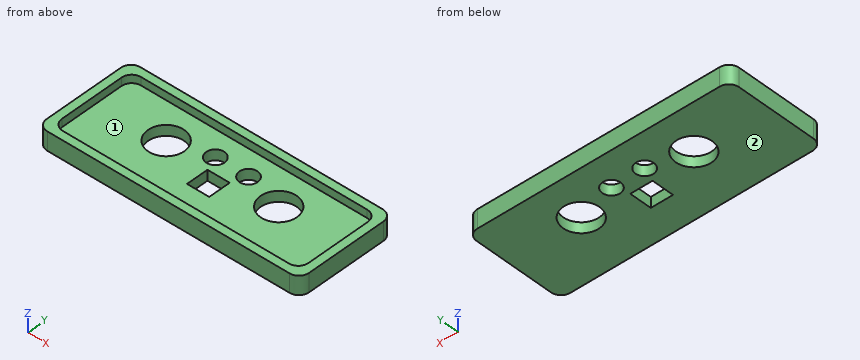
```python
from build123d import *

# Parameters (mm, degrees)
F1_DEPTH = 3.302
F2_DEPTH = 2.54
F3_R     = 5.715
F3_W     = 6.985
F3_H     = 6.985
F3_R_2   = 2.8702
F4_DEPTH = 3.303


with BuildPart() as f1:
    # F0 (on Top) → F1 (new body)
    with BuildSketch(Plane.XY):
        with BuildLine():
            Line((86.51892, -3.862933), (10.31892, -3.862933))
            ThreePointArc((10.31892, -3.862933), (8.073856, -4.792869), (7.14392, -7.037933))
            Line((7.14392, -7.037933), (7.14392, -32.437933))
            ThreePointArc((7.14392, -32.437933), (8.073856, -34.682997), (10.31892, -35.612933))
            Line((10.31892, -35.612933), (86.51892, -35.612933))
            ThreePointArc((86.51892, -35.612933), (88.763984, -34.682997), (89.69392, -32.437933))
            Line((89.69392, -32.437933), (89.69392, -7.037933))
            ThreePointArc((89.69392, -7.037933), (88.763984, -4.792869), (86.51892, -3.862933))
        make_face()
        with BuildLine():
            Line((83.97892, -33.072933), (12.85892, -33.072933))
            ThreePointArc((12.85892, -33.072933), (10.613856, -32.142997), (9.68392, -29.897933))
            Line((9.68392, -29.897933), (9.68392, -9.577933))
            ThreePointArc((9.68392, -9.577933), (10.613856, -7.332869), (12.85892, -6.402933))
            Line((12.85892, -6.402933), (83.97892, -6.402933))
            ThreePointArc((83.97892, -6.402933), (86.223984, -7.332869), (87.15392, -9.577933))
            Line((87.15392, -9.577933), (87.15392, -29.897933))
            ThreePointArc((87.15392, -29.897933), (86.223984, -32.142997), (83.97892, -33.072933))
        make_face(mode=Mode.SUBTRACT)
        with BuildLine():
            ThreePointArc((9.68392, -29.897933), (10.613856, -32.142997), (12.85892, -33.072933))
            Line((12.85892, -33.072933), (83.97892, -33.072933))
            ThreePointArc((83.97892, -33.072933), (86.223984, -32.142997), (87.15392, -29.897933))
            Line((87.15392, -29.897933), (87.15392, -9.577933))
            ThreePointArc((87.15392, -9.577933), (86.223984, -7.332869), (83.97892, -6.402933))
            Line((83.97892, -6.402933), (12.85892, -6.402933))
            ThreePointArc((12.85892, -6.402933), (10.613856, -7.332869), (9.68392, -9.577933))
            Line((9.68392, -9.577933), (9.68392, -29.897933))
        make_face()
    extrude(amount=-F1_DEPTH)

    # F0 (on Top) → F2 (join)
    with BuildSketch(Plane.XY):
        with BuildLine():
            Line((86.51892, -3.862933), (10.31892, -3.862933))
            ThreePointArc((10.31892, -3.862933), (8.073856, -4.792869), (7.14392, -7.037933))
            Line((7.14392, -7.037933), (7.14392, -32.437933))
            ThreePointArc((7.14392, -32.437933), (8.073856, -34.682997), (10.31892, -35.612933))
            Line((10.31892, -35.612933), (86.51892, -35.612933))
            ThreePointArc((86.51892, -35.612933), (88.763984, -34.682997), (89.69392, -32.437933))
            Line((89.69392, -32.437933), (89.69392, -7.037933))
            ThreePointArc((89.69392, -7.037933), (88.763984, -4.792869), (86.51892, -3.862933))
        make_face()
        with BuildLine():
            Line((83.97892, -33.072933), (12.85892, -33.072933))
            ThreePointArc((12.85892, -33.072933), (10.613856, -32.142997), (9.68392, -29.897933))
            Line((9.68392, -29.897933), (9.68392, -9.577933))
            ThreePointArc((9.68392, -9.577933), (10.613856, -7.332869), (12.85892, -6.402933))
            Line((12.85892, -6.402933), (83.97892, -6.402933))
            ThreePointArc((83.97892, -6.402933), (86.223984, -7.332869), (87.15392, -9.577933))
            Line((87.15392, -9.577933), (87.15392, -29.897933))
            ThreePointArc((87.15392, -29.897933), (86.223984, -32.142997), (83.97892, -33.072933))
        make_face(mode=Mode.SUBTRACT)
    extrude(amount=F2_DEPTH)

    # F3 (on Top) → F4 (cut, through all)
    with BuildSketch(Plane.XY):
        with Locations((30.71512, -17.197933)):
            Circle(F3_R)
        with BuildLine():
            ThreePointArc((71.83772, -17.197933), (66.12272, -11.482933), (60.40772, -17.197933))
            ThreePointArc((60.40772, -17.197933), (66.12272, -22.912933), (71.83772, -17.197933))
        make_face()
        with Locations((48.41892, -22.011233)):
            Rectangle(F3_W, F3_H)
        with Locations((43.19922, -13.949079)):
            Circle(F3_R_2)
        with BuildLine():
            ThreePointArc((56.50882, -13.949079), (53.63862, -11.078879), (50.76842, -13.949079))
            ThreePointArc((50.76842, -13.949079), (53.63862, -16.819279), (56.50882, -13.949079))
        make_face()
    extrude(amount=-F4_DEPTH, mode=Mode.SUBTRACT)


solid = f1.part
```
Geometry: final body of the model. Coordinates: model frame, mm. Face numbers are marked on the shaded views. A direction names the side the tool comes from. Give positions to 0.01 mm unless a question says otherwise; leave off trailing zeros. Loops run counter-clockwise (first coordinate to the right, second up) from the corner with the lowest first, then second, coordinate; pieces in that order, holes last. Notation, with made-up numbers: (-28.75, 46) -> (30.25, 46) arc R17 ccw to (30.25, 75) -> close; hole circle Ø1 at (10, 60.5). An arc over 180 degrees is marked (long way). Return JSON: item names as keys, results as strings.
Item 1: Pin query (flat end, axial travel): P1, Ø7.5, axis at x = 43.2, y = -13.95, coming from the +Z side. Return the tip coordinate at first contact, or that it passes through.
Filled in:
{"P1": "z = 0"}
Item 2: Section A-A, the plane x = 47. Output: boundary loops of the cut face in (y, z).
Filled in:
{"outline": "(-35.61, -3.3) -> (-25.5, -3.3) -> (-25.5, 0) -> (-33.07, 0) -> (-33.07, 2.54) -> (-35.61, 2.54) -> close; (-18.52, -3.3) -> (-3.86, -3.3) -> (-3.86, 2.54) -> (-6.4, 2.54) -> (-6.4, 0) -> (-18.52, 0) -> close"}
Item 3: Access query for the marked faces 1 and 2. Directions: +Z, -Z, +X, -X, +Y, -Y. A direction counts if a zero-diameter tool reaches every point of the face in a straight line with its end or side. Return the directions, or none.
Filled in:
{"face 1": "+Z", "face 2": "-Z, +X, -X, +Y, -Y"}
Item 4: Line query: line 1 (Y direction, x = 44, z = 0.7); line 2 (X direction, y = -22, z = -2.2); line 3 (X direction, y = -13.5, z = -0.3). Output: solid intervals per line, ascending.
Filled in:
{"line 1": "-35.61 to -33.07, -6.4 to -3.86", "line 2": "7.14 to 27.62, 33.81 to 44.93, 51.91 to 63.02, 69.22 to 89.69", "line 3": "7.14 to 26.36, 35.07 to 40.36, 46.03 to 50.8, 56.47 to 61.77, 70.48 to 89.69"}
Item 5: Section B-B, the plane y = -24.5. Output: boundary loops of the cut face in (x, z).
Filled in:
{"outline": "(7.14, -3.3) -> (44.93, -3.3) -> (44.93, 0) -> (9.68, 0) -> (9.68, 2.54) -> (7.14, 2.54) -> close; (51.91, -3.3) -> (89.69, -3.3) -> (89.69, 2.54) -> (87.15, 2.54) -> (87.15, 0) -> (51.91, 0) -> close"}
Item 6: Section C-C, the plane y = -29. Output: boundary loops of the cut face in (x, z), plus the area to 3 significant figures.
Filled in:
{"outline": "(7.14, -3.3) -> (89.69, -3.3) -> (89.69, 2.54) -> (87.15, 2.54) -> (87.15, 0) -> (9.68, 0) -> (9.68, 2.54) -> (7.14, 2.54) -> close", "area": "285 mm^2"}
Item 7: Section D-D, the plane x = 19.5. Output: boundary loops of the cut face in (y, z), plus the area to 3 significant figures.
Filled in:
{"outline": "(-35.61, -3.3) -> (-3.86, -3.3) -> (-3.86, 2.54) -> (-6.4, 2.54) -> (-6.4, 0) -> (-33.07, 0) -> (-33.07, 2.54) -> (-35.61, 2.54) -> close", "area": "118 mm^2"}
